Part model, mm, in its own coordinate system. Face numbers are marked on the shaded views. A direction names the side the tool comes from. Give positions to 0.01 mm unless a question says otherwise; leave off trailing zeros. Write each loop counter-clockwise with the first axis right and the second up, starting at its lowest first coordinate (ties: lowest second). Pieces come first, ordered by that corner, then holes.
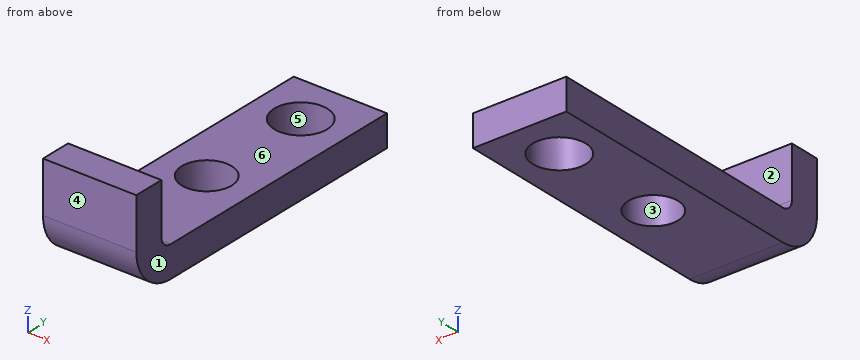
from build123d import *

# Parameters (mm, degrees)
SKETCH_1_W                       = 6
SKETCH_1_H                       = 18
SKETCH_1_R                       = 1.6
SKETCH_1_R_2                     = 1.7
SM_BASE_FLANGE_1_DEPTH           = 2
SM_EDGE_FLANGE_1_STRIP_W         = 9.4732
SM_EDGE_FLANGE_1_STRIP_H         = 2
SM_EDGE_FLANGE_1_STRIP_CUT_DEPTH = 6
SM_EDGE_FLANGE_1_DEPTH           = 6


# Sheet-metal steps are written as plain solids
with BuildPart() as part:
    # Sketch 1 → Базовая кромка1 (new body)
    with BuildSketch(Plane.XY):
        with Locations((0, 1.659676661)):
            Rectangle(SKETCH_1_W, SKETCH_1_H)
        Circle(SKETCH_1_R, mode=Mode.SUBTRACT)
        with Locations((0, 7.5)):
            Circle(SKETCH_1_R_2, mode=Mode.SUBTRACT)
    extrude(amount=-SM_BASE_FLANGE_1_DEPTH)

    # Ребро-кромка1 strip (across the edge) → Ребро-кромка1 strip cut (cut)
    with BuildSketch(Plane(origin=(-3, -7.340323339, 0), x_dir=(0, 1, 0), z_dir=(1, 0, 0))):
        with Locations((-4, -1)):
            Rectangle(SM_EDGE_FLANGE_1_STRIP_W, SM_EDGE_FLANGE_1_STRIP_H)
    extrude(amount=SM_EDGE_FLANGE_1_STRIP_CUT_DEPTH, mode=Mode.SUBTRACT)

    # Ребро-кромка1 section (across the edge) → Ребро-кромка1 (add)
    with BuildSketch(Plane(origin=(-3, -7.340323339, 0), x_dir=(0, 1, 0), z_dir=(1, 0, 0))):
        with BuildLine():
            Line((-2, 0.7366), (-2, 4))
            Line((-2, 4), (0, 4))
            Line((0, 4), (0, 0.7366))
            ThreePointArc((0, 0.7366), (0.215745145, 0.215745145), (0.7366, 0))
            Line((0.7366, 0), (0.7366, -2))
            ThreePointArc((0.7366, -2), (-1.198468417, -1.198468417), (-2, 0.7366))
        make_face()
    extrude(amount=SM_EDGE_FLANGE_1_DEPTH)


solid = part.part
1) Saw through at D-D (z = -0.2). Write the cut outline in (x, y).
Check result:
outline: (-3, -9.18) - (3, -9.18) - (3, 10.66) - (-3, 10.66) - close; hole circle Ø3.4 at (0, 7.5); hole circle Ø3.2 at (0, 0)
2) Flat gauge pins, fed straight in: P1, Ø1.6, axis at x = -1.5, z = 2, coming from the +Y side; P2, Ø1.8, axis at x = 0.5, y = 1.5, coming from the +Z side. Where does each tip first touch, or does it go through?
Check result:
P1: stops at y = -7.34
P2: stops at z = 0
3) Saw through at A-A (x = 0). Write the cut outline in (y, z), and give its area (3 significant figures).
Check result:
outline: (-9.34, 0.74) arc R2.74 ccw to (-6.6, -2) - (-1.6, -2) - (-1.6, 0) - (-6.6, 0) arc R0.74 cw to (-7.34, 0.74) - (-7.34, 4) - (-9.34, 4) - close; (1.6, -2) - (5.8, -2) - (5.8, 0) - (1.6, 0) - close; (9.2, -2) - (10.66, -2) - (10.66, 0) - (9.2, 0) - close
area: 33.3 mm2
4) 3-axis set-ups, long thin cutter, end or side, ignore diameter. For the marked faces 1 and 2: which of +Z, -Z, +X, -X, +Y, -Y reach the whole face in a straight line?
Check result:
face 1: +Z, -Z, +X, +Y, -Y
face 2: +Z, +X, -X, +Y
5) Saw through at C-C (x = -2.1). Write the cut outline in (y, z), and give its area (3 significant figures).
Check result:
outline: (-9.34, 0.74) arc R2.74 ccw to (-6.6, -2) - (10.66, -2) - (10.66, 0) - (-6.6, 0) arc R0.74 cw to (-7.34, 0.74) - (-7.34, 4) - (-9.34, 4) - close
area: 46.5 mm2
6) Saw through at B-B (y = 7.5). Write the cut outline in (x, z).
Check result:
outline: (-3, -2) - (-1.7, -2) - (-1.7, 0) - (-3, 0) - close; (1.7, -2) - (3, -2) - (3, 0) - (1.7, 0) - close
7) Mould opens along Y. For the marked faces 3, 4, 5 and 6 say: +Y half, -Y half, draft (parallel to the pull), parting line (faces both ways), or undercut.
Check result:
face 3: undercut
face 4: -Y half
face 5: undercut
face 6: draft
8) Drill centre lines: L1, parallel to Y at x = -0.7, z = -1.55; L2, parallel to Y at x = 0, z = -1; L3, parallel to Z at x = 1.2, y = 10.25. Where is each one in solid material? Low to high.
Check result:
L1: y = -8.11 to -1.44, 1.44 to 5.95, 9.05 to 10.66
L2: y = -8.72 to -1.6, 1.6 to 5.8, 9.2 to 10.66
L3: z = -2 to 0
